Autodesk Fusion 360 part; units mm, degrees
sketch "Sketch1" plane through (0, 0, 0) normal (0, 0, 1) x (1, 0, 0)
  line L0 (-90, 75) -> (180, 75)
  line L1 (190, 65) -> (190, -475)
  line L2 (180, -485) -> (-90, -485)
  line L3 (-100, -475) -> (-100, 65)
  line L4 (170, -475) -> (-80, -475)
  line L5 (-90, -465) -> (-90, 55)
  line L6 (-80, 65) -> (170, 65)
  line L7 (180, 55) -> (180, -465)
  arc A0 (190, 65) -> (180, 75) centre (180, 65) ccw
  arc A1 (180, 55) -> (170, 65) centre (170, 55) ccw
  arc A2 (-80, 65) -> (-90, 55) centre (-80, 55) ccw
  arc A3 (180, -485) -> (190, -475) centre (180, -475) ccw
  arc A4 (-90, 75) -> (-100, 65) centre (-90, 65) ccw
  arc A5 (170, -475) -> (180, -465) centre (170, -465) ccw
  arc A6 (-90, -465) -> (-80, -475) centre (-80, -465) ccw
  arc A7 (-100, -475) -> (-90, -485) centre (-90, -475) ccw
  point P0 (-100, 75)
  point P1 (190, 75)
  point P2 (-100, -485)
  dimension "d1" = 290
  dimension "d2" = 560
  dimension "d4" = 10
  dimension "d5" = 10
extrude "Extrude1" add sketch "Sketch1" along normal blind 100
extrude "Extrude2" add sketch "Sketch1" along normal blind 20 contours L4 L5 L6 L7 A1 A2 A5 A6
sketch "Sketch2" plane through (-100, 0, 0) normal (-1, 0, 0) x (0, -1, 0)
  line L0 (-65, 0) -> (475, 0)
  line L1 (475, 0) -> (475, 100)
  line L2 (475, 100) -> (-65, 100)
  line L3 (-65, 100) -> (-65, 0)
  line L4 (160, 79.717) -> (236.5175, 79.717)
  arc A0 (236.5175, 79.717) -> (236.5175, 100.283) centre (236.5175, 90) ccw
  line L5 (236.5175, 100.283) -> (160, 100.283)
  arc A1 (160, 100.283) -> (160, 79.717) centre (160, 90) ccw
  line L6 (160, 90) -> (236.5175, 90) construction
extrude "Extrude3" cut sketch "Sketch2" against normal blind 40 contours L2 L4 A0 A1
Read the model definition and answer for the solid it produces. Units are mm, in the model's axes. A direction names the side the tool comes from. Coordinates: 2 decimals unless noted, no trailing zeros. Loops run counter-clockwise (first coordinate to the right, second up) from the corner with the lowest first, then second, coordinate; pieces in that order, holes last.
Q1. Consider probe 1 along Y at (x, z) = (168.5, 46); probe 2 along X at (y, z) = (-342, 60); probe 3 along Z at (x, y) = (-86, -8.5). Determine where each line is inside the solid, lowest interval first.
Q2. The part is cut by section C-C on y = -378.5. Write down the section's boundary in (x, z).
Q3. The part is cut by section A-A on x = 31. Write down the section's boundary in (y, z), and give its area (3 significant figures).
Q4. Each of these flat-tipped pins is pushed along its axis until it touches: pin 1 Ø3 at (y, z) = (-224, 87.5) entering from -X; pin 2 Ø1.5 at (x, y) = (132, -268) entering from +Z; pin 3 Ø8 at (x, y) = (-93, -201) entering from +Z. Where does it stop, or does it pass through?
Q5. The part is cut by section B-B on z = 66.5. Write down the section's boundary in (x, y), and give its area (3 significant figures).
Q6. Which of the six approach directions +Z, -Z, +X, -X, +Y, -Y give full straight-line access (tool end or side, diameter ignored) to faces 4 (the face through (177.15, -471.99, 59.44)), 5 (the face through (-95, -198, 79.717)), 6 (the face through (-95.07, -149.766, 89.002))?
Q7. The mould has two halves that part along Y. Classify faces 1 (the face through (190, -201, 49)), 2 (the face through (-86.99, -472.15, 59.44)), 3 (the face through (-96.99, -482.15, 49.3)): +Y half, -Y half, draft (parallel to the pull), parting line (faces both ways), or undercut.
Results below:
1. probe 1: y = -485 to -475, 65 to 75
1. probe 2: x = -100 to -90, 180 to 190
1. probe 3: z = 0 to 20
2. outline: (-100, 0) - (190, 0) - (190, 100) - (180, 100) - (180, 20) - (-90, 20) - (-90, 100) - (-100, 100) - close
3. outline: (-485, 0) - (75, 0) - (75, 100) - (65, 100) - (65, 20) - (-475, 20) - (-475, 100) - (-485, 100) - close
3. area: 12,800 mm2
4. pin 1: stops at x = 180
4. pin 2: stops at z = 20
4. pin 3: stops at z = 79.72
5. outline: (-100, -475) arc R10 ccw to (-90, -485) - (180, -485) arc R10 ccw to (190, -475) - (190, 65) arc R10 ccw to (180, 75) - (-90, 75) arc R10 ccw to (-100, 65) - close; hole (-90, -465) arc R10 ccw to (-80, -475) - (170, -475) arc R10 ccw to (180, -465) - (180, 55) arc R10 ccw to (170, 65) - (-80, 65) arc R10 ccw to (-90, 55) - close
5. area: 16,600 mm2
6. face 4: +Z
6. face 5: +Z, -X
6. face 6: -X
7. face 1: draft
7. face 2: undercut
7. face 3: -Y half
